Build history of the part. All positions in model axes, mm. A direction names the side the tool comes from. Give positions to 0.01 mm unless a question says otherwise; leave off trailing zeros. Loops run counter-clockwise (first coordinate to the right, second up) from the corner with the lowest first, then second, coordinate; pieces in that order, holes last. Notation, with made-up numbers: M 87,24 L 115,24 A26 ccw 115,44 Z; hole C 70,33.5 d4. An arc over 180 degrees is marked long. Answer as a JSON object with one key per item and string values. Group by question number.
1. Slice it at C-C (y = 1). List the corners of the cut face in (x, z).
2. Drop flat-ended pins along their axis: pin 1 Ø2 at (y, z) = (5, 11.5) entering from -X; pin 2 Ø1 at (x, z) = (-4.5, -14) entering from -Y; pin 3 Ø6.5 at (x, z) = (0, 0) entering from +Y. Give the stop position or say it passes through.
3. Slice it at D-D (x = -5.5). List the corners of the cut face in (y, z), then the cut area to 3 significant figures.
4. Slice it at A-A (x = 0). List the corners of the cut face in (y, z).
5. Slice it at B-B (z = 0). List the corners of the cut face in (x, y).
6. Drill centre lines: line 1 along Z through (x, y) = (0, 5.9); line 2 along X through (y, z) = (4.45, 0). Where is each one in solid material? Low to high. Write a range as [from, to].
7. 3-axis set-ups, long thin cutter, end or side, ignore diameter. For faces 4 (the face through (-0.867, 5.141, 3.905)), 5 (the face through (1, -0.65, -4)), 6 (the face through (2, 0.2, 0)): which of +Z, -Z, +X, -X, +Y, -Y reach the whole face in a straight line?
8. Mould opens along Z. For faces 1 (the face through (-1.42, 8, 3.92)), 2 (the face through (-1.02, -0.32, -4.59)), 3 (the face through (-0.83, -0.23, -3.76)) say: released by +Z, released by -Z, zero draft, split by the parting line, or undercut.
from build123d import *

# Parameters (mm, degrees)
SKETCH_1_R          = 19.75
EXTRUDE_1_DEPTH     = 5
SKETCH_2_R          = 6
EXTRUDE_2_DEPTH     = 3
SKETCH_3_R          = 4.7
EXTRUDE_3_DEPTH     = 0.65
SKETCH_4_R          = 1.6
CUT_EXTRUDE_1_DEPTH = 9.65
SKETCH_5_R          = 3.85
CUT_EXTRUDE_2_DEPTH = 0.85
SKETCH_6_R          = 4
CUT_EXTRUDE_3_DEPTH = 5.8


with BuildPart() as part:
    # 草圖1 → 填料-伸長1 (new body)
    with BuildSketch(Plane(origin=(0, 0, 0), x_dir=(1, 0, 0), z_dir=(0, 1, 0))):
        Circle(SKETCH_1_R)
    extrude(amount=EXTRUDE_1_DEPTH)

    # 草圖2 → 填料-伸長2 (add)
    with BuildSketch(Plane(origin=(0, 5, 0), x_dir=(1, 0, 0), z_dir=(0, 1, 0))):
        Circle(SKETCH_2_R)
    extrude(amount=EXTRUDE_2_DEPTH)

    # 草圖3 → 填料-伸長3 (add)
    with BuildSketch(Plane.XZ):
        Circle(SKETCH_3_R)
    extrude(amount=EXTRUDE_3_DEPTH)

    # 草圖4 → 除料-伸長1 (cut, through all)
    with BuildSketch(Plane.XZ.offset(0.65)):
        Circle(SKETCH_4_R)
    extrude(amount=-CUT_EXTRUDE_1_DEPTH, mode=Mode.SUBTRACT)

    # 草圖5 → 除料-伸長2 (cut)
    with BuildSketch(Plane.XZ.offset(0.65)):
        Circle(SKETCH_5_R)
    extrude(amount=-CUT_EXTRUDE_2_DEPTH, mode=Mode.SUBTRACT)

    # 草圖6 → 除料-伸長3 (cut)
    with BuildSketch(Plane(origin=(0, 8, 0), x_dir=(1, 0, 0), z_dir=(0, 1, 0))):
        Circle(SKETCH_6_R)
    extrude(amount=-CUT_EXTRUDE_3_DEPTH, mode=Mode.SUBTRACT)


solid = part.part
Established:
{
 "1": {"outline": "C 0,0 d39.5; hole C 0,0 d3.2"},
 "2": {"pin 1": "stops at x = -16.73", "pin 2": "stops at y = 0", "pin 3": "stops at y = 2.2"},
 "3": {"outline": "M 0,-18.97 L 5,-18.97 L 5,-2.4 L 8,-2.4 L 8,2.4 L 5,2.4 L 5,18.97 L 0,18.97 Z", "area": "204 mm^2"},
 "4": {"outline": "M -0.65,-4.7 L 0,-4.7 L 0,-19.75 L 5,-19.75 L 5,-6 L 8,-6 L 8,-4 L 2.2,-4 L 2.2,-1.6 L 0.2,-1.6 L 0.2,-3.85 L -0.65,-3.85 Z; M -0.65,3.85 L 0.2,3.85 L 0.2,1.6 L 2.2,1.6 L 2.2,4 L 8,4 L 8,6 L 5,6 L 5,19.75 L 0,19.75 L 0,4.7 L -0.65,4.7 Z"},
 "5": {"outline": "M -19.75,0 L -4.7,0 L -4.7,-0.65 L -3.85,-0.65 L -3.85,0.2 L -1.6,0.2 L -1.6,2.2 L -4,2.2 L -4,8 L -6,8 L -6,5 L -19.75,5 Z; M 1.6,0.2 L 3.85,0.2 L 3.85,-0.65 L 4.7,-0.65 L 4.7,0 L 19.75,0 L 19.75,5 L 6,5 L 6,8 L 4,8 L 4,2.2 L 1.6,2.2 Z"},
 "6": {"line 1": "z = [-6, -4], [4, 6]", "line 2": "x = [-19.75, -4], [4, 19.75]"},
 "7": {"face 4": "+Y", "face 5": "+Z, -Z, +X, -X, -Y", "face 6": "-Y"},
 "8": {"face 1": "zero draft", "face 2": "split by the parting line", "face 3": "undercut"}
}
